CAD build for the part. Positions are in the model's coordinates, mm. Round coordinates to 2 decimals unless told otherwise and drop trailing zeros. Loops run counter-clockwise (first coordinate to the right, second up) from the corner with the lowest first, then second, coordinate; pieces in that order, holes last.
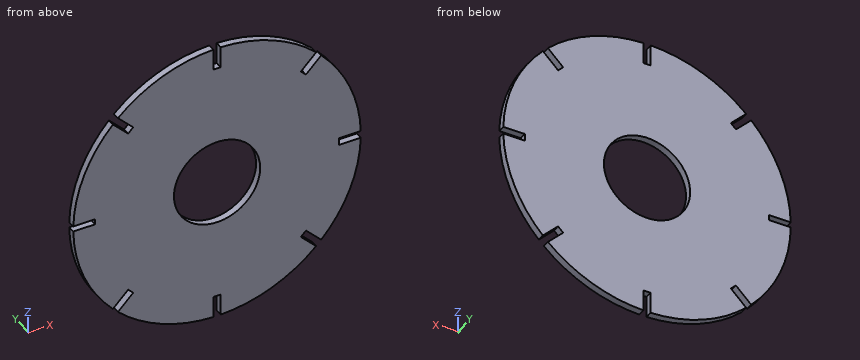
```python
from build123d import *

# Parameters (mm, degrees)
F0_R     = 38.1
F1_DEPTH = 6.35
F3_DEPTH = 25.4


with BuildPart() as f1:
    # F0 (on Front) → F1 (new body)
    with BuildSketch(Plane.XZ):
        with BuildLine():
            Line((107.910306, 3.175), (126.960306, 3.175))
            ThreePointArc((126.960306, 3.175), (89.802561, 89.802561), (3.175, 126.960306))
            Line((3.175, 126.960306), (3.175, 107.95))
            Line((3.175, 107.95), (-3.175, 107.95))
            Line((-3.175, 107.95), (-3.175, 126.960306))
            ThreePointArc((-3.175, 126.960306), (-89.802561, 89.802561), (-126.960306, 3.175))
            Line((-126.960306, 3.175), (-107.910306, 3.175))
            Line((-107.910306, 3.175), (-107.910306, -1.5875))
            Line((-107.910306, -1.5875), (-126.990078, -1.5875))
            ThreePointArc((-126.990078, -1.5875), (-90.362171, -89.239442), (-3.175, -126.960306))
            Line((-3.175, -126.960306), (-3.175, -107.910306))
            Line((-3.175, -107.910306), (3.175, -107.910306))
            Line((3.175, -107.910306), (3.175, -126.960306))
            ThreePointArc((3.175, -126.960306), (89.802561, -89.802561), (126.960306, -3.175))
            Line((126.960306, -3.175), (107.910306, -3.175))
            Line((107.910306, -3.175), (107.910306, 3.175))
        make_face()
        Circle(F0_R, mode=Mode.SUBTRACT)
    extrude(amount=F1_DEPTH)

    # F2 (on face) → F3 (cut)
    with BuildSketch(Plane.XZ.offset(6.35)):
        Polygon((74.059045, 78.549173), (76.304109, 76.304109), (78.549173, 74.059045), (92.019558, 87.529429), (97.280774, 92.737254), (92.76395, 97.254078), (87.529429, 92.019558), align=None)
        Polygon((78.549173, -74.059045), (76.304109, -76.304109), (74.059045, -78.549173), (87.529429, -92.019558), (97.125031, -102.679037), (102.767334, -97.599868), (92.019558, -87.529429), align=None)
        Polygon((-74.059045, -78.549173), (-76.304109, -76.304109), (-78.549173, -74.059045), (-92.019558, -87.529429), (-97.248051, -92.726782), (-92.600375, -97.240731), (-87.529429, -92.019558), align=None)
        Polygon((-78.549173, 74.059045), (-76.304109, 76.304109), (-74.059045, 78.549173), (-87.529429, 92.019558), (-93.063728, 97.553856), (-97.69151, 92.926074), (-92.019558, 87.529429), align=None)
    extrude(amount=-F3_DEPTH, mode=Mode.SUBTRACT)


solid = f1.part
```
Item 1: Flat gauge pins, fed straight in: P1, Ø3, axis at y = -4.5, z = 0, coming from the +X side; P2, Ø10, axis at x = -78, z = -34, coming from the +Y side; P3, Ø1.9, axis at x = 116, y = -4.5, coming from the -Z side; P4, Ø3, axis at y = -4.5, z = 37, coming from the +X side. Where does each tip first touch, or does it go through?
Answers follow:
P1: stops at x = 107.91
P2: stops at y = 0
P3: stops at z = -53.78
P4: stops at x = 121.94
Item 2: Cut at D-D, the plane x = 41. Give the cut face in (y, z), plus the area to 3 significant figures.
Answers follow:
outline: (-6.35, -120.2) - (0, -120.2) - (0, 120.2) - (-6.35, 120.2) - close
area: 1,530 mm2
Item 3: Probe line 1 (X direction, y = -3.25, z = -86); line 2 (Z direction, x = 1, y = -6); line 3 (X direction, y = -0.5, z = 112.5) (3 decimals). List the from-to ranges inside material, lowest first.
Answers follow:
line 1: x = -93.45 to -90.49, -81.51 to 81.51, 90.49 to 93.45
line 2: z = -107.91 to -38.09, 38.09 to 107.95
line 3: x = -58.93 to -3.175, 3.175 to 58.93
Item 4: Cut at B-B, the plane x = 0. Give the cut face in (y, z), plus the area to 3 significant figures.
Answers follow:
outline: (-6.35, -107.91) - (0, -107.91) - (0, -38.1) - (-6.35, -38.1) - close; (-6.35, 38.1) - (0, 38.1) - (0, 107.95) - (-6.35, 107.95) - close
area: 887 mm2
Item 5: Cut at C-C, the plane z = 21. Give the cut face in (x, y), plus the area to 3 significant figures.
Answers follow:
outline: (-125.25, -6.35) - (-31.79, -6.35) - (-31.79, 0) - (-125.25, 0) - close; (31.79, -6.35) - (125.25, -6.35) - (125.25, 0) - (31.79, 0) - close
area: 1,190 mm2
